For this review, take the finished solid that the model builds, in its own axes (mm). A direction names the side the tool comes from. Round coordinates to 2 decimals unless told otherwise and drop trailing zeros. Write each loop counter-clockwise with the first axis right and the second up, starting at its lowest first coordinate (ties: lowest second). Pieces come first, ordered by that corner, then holes. Notation, with made-up numbers: M 5.25,-15.5 L 21.25,-15.5 A23 cw 21.25,18.5 Z; hole C 61,88 d8. An arc over 180 degrees is marked long. Answer in a Markdown table with one row per item.
```python
from build123d import *

# Parameters (mm, degrees)
SKETCH_R        = 7.9375
PAD_DEPTH       = 31.7
SKETCH001_W     = 4.76
SKETCH001_H     = 4.76
PAD001_DEPTH    = 25
SKETCH002_R     = 41.275
PAD002_DEPTH    = 6.4
SKETCH003_R     = 5.55
PAD003_DEPTH    = 8
PAD004_DEPTH    = 142.6
SKETCH005_R     = 12.7
POCKET_DEPTH    = 12.7
SKETCH006_R     = 10.16
PAD005_DEPTH    = 35
SKETCH007_R     = 9.525
POCKET001_DEPTH = 12.7


with BuildPart() as part:
    # Sketch → Pad (new body)
    with BuildSketch(Plane.XY):
        Circle(SKETCH_R)
    extrude(amount=PAD_DEPTH)

    # Sketch001 → Pad001 (new body)
    with BuildSketch(Plane(origin=(0, 0, 0), x_dir=(1, 0, 0), z_dir=(0, 0, -1))):
        with Locations((0, 7.9375)):
            Rectangle(SKETCH001_W, SKETCH001_H)
    extrude(amount=-PAD001_DEPTH)

    # Sketch002 → Pad002 (new body)
    with BuildSketch(Plane.XY.offset(31.7)):
        Circle(SKETCH002_R)
    extrude(amount=PAD002_DEPTH)

    # Sketch003 → Pad003 (new body)
    with BuildSketch(Plane.XY.offset(38.1)):
        with BuildLine():
            Line((-64.75, 12.806207), (-64.75, -12.806207))
            Line((-64.75, -12.806207), (-19.05, -40.76883))
            ThreePointArc((-19.05, -40.76883), (0, -45), (19.05, -40.76883))
            Line((19.05, -40.76883), (64.75, -12.806207))
            Line((64.75, 12.806207), (64.75, -12.806207))
            Line((19.05, 40.76883), (64.75, 12.806207))
            ThreePointArc((19.05, 40.76883), (0, 45), (-19.05, 40.76883))
            Line((-64.75, 12.806207), (-19.05, 40.76883))
        make_face()
        with Locations((-53.2, 0)):
            Circle(SKETCH003_R, mode=Mode.SUBTRACT)
        with Locations((53.2, 0)):
            Circle(SKETCH003_R, mode=Mode.SUBTRACT)
    extrude(amount=PAD003_DEPTH)

    # Sketch004 → Pad004 (new body)
    with BuildSketch(Plane.XY.offset(46.1)):
        with BuildLine():
            Line((-45, 10), (-45, -40.8))
            ThreePointArc((-45, -40.8), (-39.107056, -55.772577), (-25.4, -64.2))
            Line((-25.4, -64.2), (25.4, -64.2))
            ThreePointArc((25.4, -64.2), (39.107056, -55.772577), (45, -40.8))
            Line((45, 10), (45, -40.8))
            ThreePointArc((45, 10), (37.218977, 20.269607), (25.4, 25.4))
            Line((-25.4, 25.4), (25.4, 25.4))
            ThreePointArc((-25.4, 25.4), (-37.218977, 20.269607), (-45, 10))
        make_face()
    extrude(amount=PAD004_DEPTH)

    # Sketch005 → Pocket (cut)
    with BuildSketch(Plane.YZ.offset(45)):
        with Locations((-12.7, 117.7)):
            Circle(SKETCH005_R)
    extrude(amount=-POCKET_DEPTH, mode=Mode.SUBTRACT)

    # Sketch006 → Pad005 (new body)
    with BuildSketch(Plane.YZ.offset(45)):
        with Locations((-10.16, 84.2)):
            Circle(SKETCH006_R)
    extrude(amount=PAD005_DEPTH)

    # Sketch007 → Pocket001 (cut)
    with BuildSketch(Plane(origin=(-45, 0, 0), x_dir=(0, -1, 0), z_dir=(-1, 0, 0))):
        with Locations((9.525, 164.2)):
            Circle(SKETCH007_R)
    extrude(amount=-POCKET001_DEPTH, mode=Mode.SUBTRACT)


solid = part.part
```
Q1. Take a section at C-C (x = -53.2). State the section outline as (y, z) points, then the cut area to 3 significant figures.
Found:
| item | result |
|---|---|
| outline | M -19.87,38.1 L -5.55,38.1 L -5.55,46.1 L -19.87,46.1 Z; M 5.55,38.1 L 19.87,38.1 L 19.87,46.1 L 5.55,46.1 Z |
| area | 229 mm² |
Q2. For probe 1 along Z at (x, y) = (41, -12); probe 2 along X at (y, z) = (-2.5, 149.5); probe 3 along Z at (x, y) = (44.5, -29.5), list the stretches that pass through material, from the lowest coordinate up.
Found:
| item | result |
|---|---|
| probe 1 | 38.1 to 105.02, 130.38 to 188.7 |
| probe 2 | -45 to 45 |
| probe 3 | 46.1 to 188.7 |
Q3. Take a section at D-D (z = 117.7). State the section outline as (x, y) points.
Found:
| item | result |
|---|---|
| outline | M -45,-40.8 A25.4 ccw -25.4,-64.2 L 25.4,-64.2 A25.4 ccw 45,-40.8 L 45,-25.4 L 32.3,-25.4 L 32.3,0 L 45,0 L 45,10 A25.4 ccw 25.4,25.4 L -25.4,25.4 A25.4 ccw -45,10 Z |
Q4. Mouldability with a two-part tool opening along Z and no side actions: class faces 1 (the face through (39, -55.9, 116.4)), 2 (the face through (-1, -19, 188.7)), 3 (the face through (38.739, -14.353, 130.292)) as +Z half, -Z half, draft (parallel to the pull), parting line (faces both ways), or undercut.
Found:
| item | result |
|---|---|
| face 1 | draft |
| face 2 | +Z half |
| face 3 | undercut |
Q5. Take a section at B-B (x = 0). State the section outline as (y, z) points (1 decimal).
Found:
| item | result |
|---|---|
| outline | M -64.2,46.1 L -45,46.1 L -45,38.1 L -41.3,38.1 L -41.3,31.7 L -7.9,31.7 L -7.9,25 L -10.3,25 L -10.3,0 L 7.9,0 L 7.9,31.7 L 41.3,31.7 L 41.3,38.1 L 45,38.1 L 45,46.1 L 25.4,46.1 L 25.4,188.7 L -64.2,188.7 Z |
Q6. Take a section at A-A (z = 149). State the section outline as (x, y) points.
Found:
| item | result |
|---|---|
| outline | M -45,-40.8 A25.4 ccw -25.4,-64.2 L 25.4,-64.2 A25.4 ccw 45,-40.8 L 45,10 A25.4 ccw 25.4,25.4 L -25.4,25.4 A25.4 ccw -45,10 Z |
Q7. Machinability: for faces 4 (the face through (32.3, -13, 118)), 5 (the face through (0, 25.4, 116)), 6 (the face through (58.327, -2.126, 42.044)), 7 (the face through (-32.3, -9, 164)), 8 (the face through (41.58, -26.983, 42.044)), which of the approach directions +Z, -Z, +X, -X, +Y, -Y give a long, thin tool a straight path to every point of the face, cutting with its end or side? Answer none if there is none.
Found:
| item | result |
|---|---|
| face 4 | +X |
| face 5 | +Z, +X, -X, +Y |
| face 6 | -Z |
| face 7 | -X |
| face 8 | -Z, +X, -Y |
Q8. Insertion check: P1, Ø4, axis at y = 4.5, z = 43, coming from the +X side; P2, Ø3, axis at x = 7, z = 112.5, coming from the +Y side; P3, Ø20.5, axis at y = -12.7, z = 117.7, coming from the -X side. Each pin has a flat end and moves straight along its axis. Give the tip position at first contact, or say it passes through.
Found:
| item | result |
|---|---|
| P1 | x = 64.75 |
| P2 | y = 25.4 |
| P3 | x = -45 |
